Part print with two shaded views. Sizes in mm from the minimum x, y, z corner. Coordinates: 2 decimals unless noted, no trailing zeros. Order: outer loops, then holes, each group sorted by start corner. A loop starts at its lowest first (then second) coordinate and runs counter-clockwise, first axis right, second up. Notation, with made-up numbers: (-40, -40) - (9, -40) arc R7 cw to (9, -35) - close; hole circle Ø6 at (53, -21). An arc over 180 degrees is marked (long way). Write each question's results on one line, items separated by ' | '. Start each with the question number.
Q1. Band-saw the part on A-A, the plane z = 65. Write the cut outline in (x, y) (3 decimals), then the cut area to 3 significant figures.
Q2. Pin check, flat tip, straight feed: P1, Ø2.5, axis at x = 15, z = 35, coming from the +Y side (3 decimals). Stop position of the tip, or through.
Q3. Wall check: probe 1 along X at (y, z) = (1.4, 15); probe 2 along X at (y, z) = (2.45, 75.5); probe 3 along Z at (x, y) = (28.5, 2.3). Give the ranges that are in metal, low to high.
Q4. Band-saw the part on B-B, the plane y = 1.9. Count the separate pieces of the cut face and the enclosed holes in it, then the cut area to 3 significant figures.
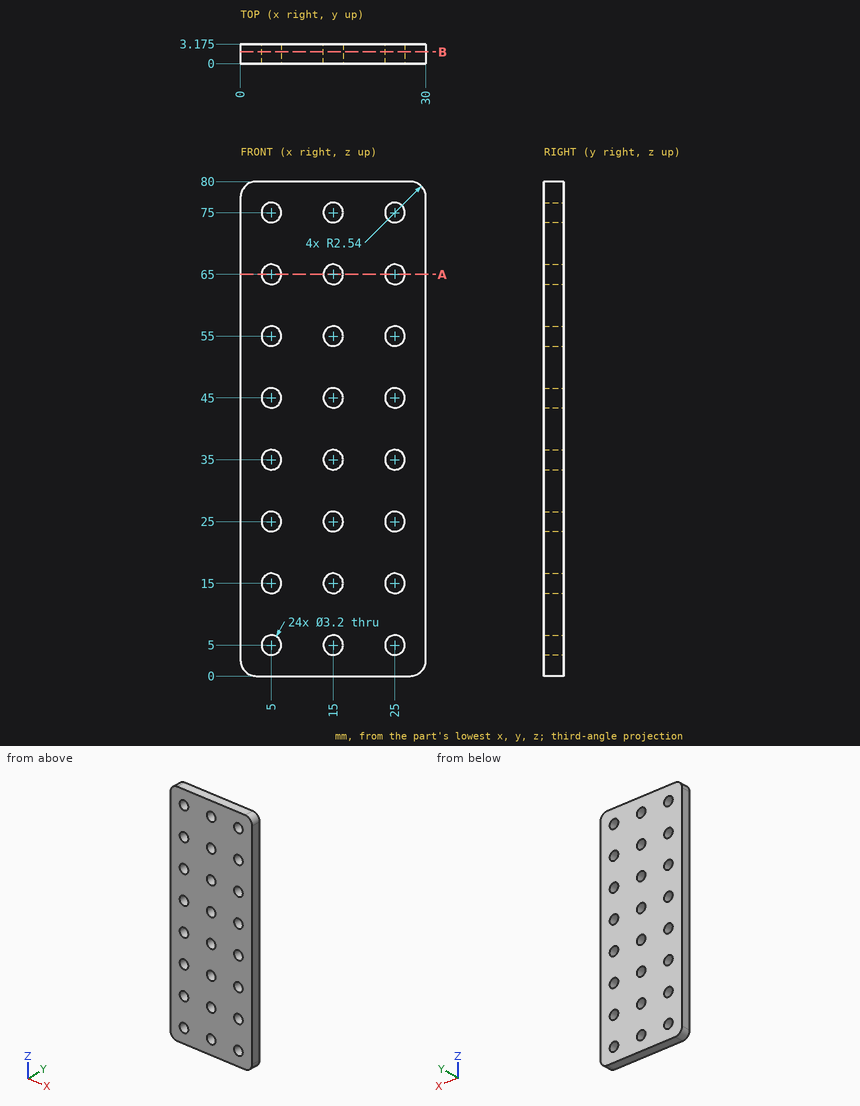
Results below:
1) outline: (0, 0) - (3.4, 0) - (3.4, 3.175) - (0, 3.175) - close; (6.6, 0) - (13.4, 0) - (13.4, 3.175) - (6.6, 3.175) - close; (16.6, 0) - (23.4, 0) - (23.4, 3.175) - (16.6, 3.175) - close; (26.6, 0) - (30, 0) - (30, 3.175) - (26.6, 3.175) - close | area: 64.8 mm²
2) P1: passes through
3) probe 1: x = 0 to 3.4, 6.6 to 13.4, 16.6 to 23.4, 26.6 to 30 | probe 2: x = 0 to 3.48, 6.52 to 13.48, 16.52 to 23.48, 26.52 to 30 | probe 3: z = 0.22 to 79.78
4) separate pieces: 1 | enclosed holes: 24 | area: 2,200 mm²
